Print and shaded views of the part. All mm, measured from the part's lowest x, y and z. A direction names the side the tool comes from. Give positions to 0.01 mm unless a question says otherwise; leave off trailing zeros. Order: outer loops, then holes, each group sorted by start corner. A loop starts at its lowest first (then second) coordinate and runs counter-clockwise, first axis right, second up. Notation, with made-up numbers: (-4.5, 67.25) -> (51.5, 67.25) arc R29 cw to (51.5, 101.25) -> close; hole circle Ø9 at (-26.75, 47). An arc over 180 degrees is marked (long way). One line per question, with ' | ' between items. Start each with the question number.
(1) Cut at A-A (x = 10.5). Give the cut face in (y, z), then the cut area to 3 significant figures.
(2) Cut at D-D (y = 4.85). Give the cut face in (x, z), then the cut area to 3 significant figures.
(3) Cut at C-C (y = 0.6). Give the cut face in (x, z).
(4) Pin check, flat tips, straight feed: pin 1 Ø3 at (x, y) = (4.5, 4) entering from -Z; pin 2 Ø2 at (x, y) = (17, 5) entering from -Z. Stop position of each tip, or through.
(5) Drill centre lines: L1, parallel to X at y = 1.35, z = 10.5; L2, parallel to Y at x = 10.75, z = 10. Where is each one in solid material? Low to high. Write a range as from..to.
(6) Cut at B-B (z = 10.5). Give the cut face in (x, y), then the cut area to 3 significant figures.
(7) Pull direction Z, two halves, no side cores. Call the marked faces 3, 4 and 5: +Z half, -Z half, draft (parallel to the pull), parting line (faces both ways), or undercut.
(8) Which spindle directions (+Z, -Z, +X, -X, +Y, -Y) get a long thin tool onto all of the face, cutting with end or side? Do the marked faces 1 and 2. Say none if no direction does.
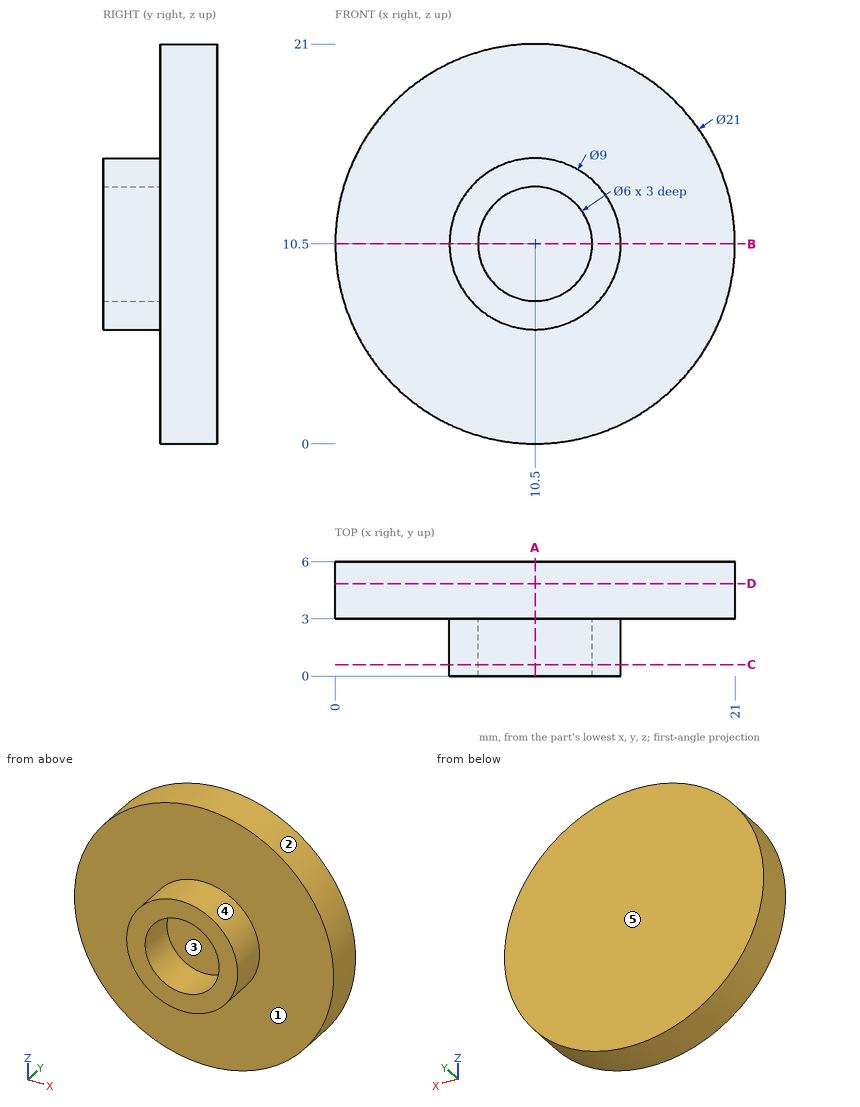
Result set:
1) outline: (0, 6) -> (3, 6) -> (3, 0) -> (6, 0) -> (6, 21) -> (3, 21) -> (3, 15) -> (0, 15) -> (0, 13.5) -> (3, 13.5) -> (3, 7.5) -> (0, 7.5) -> close | area: 72.0 mm2
2) outline: circle Ø21 at (10.5, 10.5) | area: 346 mm2
3) outline: circle Ø9 at (10.5, 10.5); hole circle Ø6 at (10.5, 10.5)
4) pin 1: stops at z = 1.01 | pin 2: stops at z = 1.56
5) L1: x = 6..7.5, 13.5..15 | L2: y = 3..6
6) outline: (0, 3) -> (6, 3) -> (6, 0) -> (7.5, 0) -> (7.5, 3) -> (13.5, 3) -> (13.5, 0) -> (15, 0) -> (15, 3) -> (21, 3) -> (21, 6) -> (0, 6) -> close | area: 72.0 mm2
7) face 3: undercut | face 4: parting line | face 5: draft
8) face 1: -Y | face 2: +Y, -Y
